```python
from build123d import *

# Parameters (mm, degrees)
ESQUISSE1_W             = 478.153686012
ESQUISSE1_H             = 188.593708553
ESQUISSE1_R             = 4
BOSS_EXTRU_4_DEPTH      = 5
ESQUISSE2_W             = 35.2
ESQUISSE2_H             = 34
ESQUISSE2_W_2           = 11
ENL_V_MAT_EXTRU_1_DEPTH = 2


with BuildPart() as part:
    # Esquisse1 → Boss.-Extru.4 (new body)
    with BuildSketch(Plane(origin=(0, 0, 0), x_dir=(1, 0, 0), z_dir=(0, 1, 0))):
        with Locations((166.159297522, 47.085285911)):
            Rectangle(ESQUISSE1_W, ESQUISSE1_H)
        with Locations(Location((395.236140528, -37.211568366, 0), (0, 0, 270))):
            Circle(ESQUISSE1_R, mode=Mode.SUBTRACT)
        with Locations(Location((-62.917545484, -37.211568366, 0), (0, 0, 270))):
            Circle(ESQUISSE1_R, mode=Mode.SUBTRACT)
        with Locations(Location((-32.917545484, -37.211568366, 0), (0, 0, 270))):
            Circle(ESQUISSE1_R, mode=Mode.SUBTRACT)
        with Locations(Location((365.236140528, -37.211568366, 0), (0, 0, 270))):
            Circle(ESQUISSE1_R, mode=Mode.SUBTRACT)
        with Locations(Location((-62.917545484, 131.382140187, 0), (0, 0, 270))):
            Circle(ESQUISSE1_R, mode=Mode.SUBTRACT)
        with Locations(Location((-32.917545484, 131.382140187, 0), (0, 0, 270))):
            Circle(ESQUISSE1_R, mode=Mode.SUBTRACT)
        with Locations(Location((365.236140528, 131.382140187, 0), (0, 0, 270))):
            Circle(ESQUISSE1_R, mode=Mode.SUBTRACT)
        with Locations(Location((395.236140528, 131.382140187, 0), (0, 0, 270))):
            Circle(ESQUISSE1_R, mode=Mode.SUBTRACT)
    extrude(amount=BOSS_EXTRU_4_DEPTH)

    # Esquisse2 → Enlèv. mat.-Extru.1 (cut)
    with BuildSketch(Plane(origin=(0, 5, 0), x_dir=(1, 0, 0), z_dir=(0, 1, 0))):
        with Locations((148.559297522, 122.382140187)):
            Rectangle(ESQUISSE2_W, ESQUISSE2_H)
        with Locations((171.659297522, 122.382140187)):
            Rectangle(ESQUISSE2_W_2, ESQUISSE2_H)
        with Locations((148.559297522, -28.211568366)):
            Rectangle(ESQUISSE2_W, ESQUISSE2_H)
        with Locations((171.659297522, -28.211568366)):
            Rectangle(ESQUISSE2_W_2, ESQUISSE2_H)
    extrude(amount=-ENL_V_MAT_EXTRU_1_DEPTH, mode=Mode.SUBTRACT)


solid = part.part
```
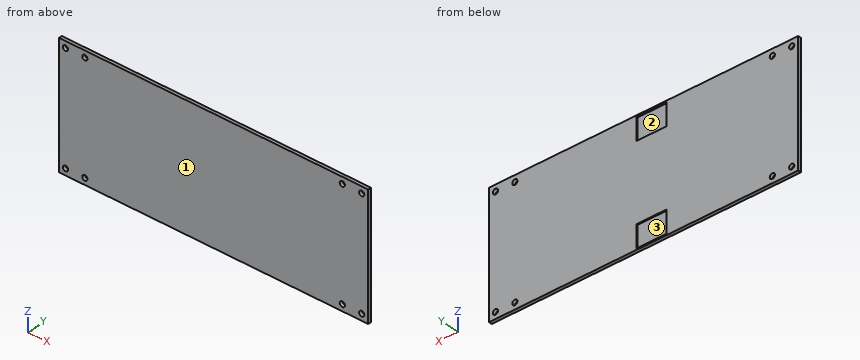
Here's how the part is built. I have some questions about the finished solid (model axes, mm). Face numbers are marked on the shaded views. Round coordinates to 2 decimals unless told otherwise and drop trailing zeros. Loops run counter-clockwise (first coordinate to the right, second up) from the corner with the lowest first, then second, coordinate; pieces in that order, holes last.
1. Will this pin go through, and if not, where does the flat tip stop? pin 1 (17 mm diameter, centred on x = 159.5, z = 35, fed in from +Y).
Answers:
pin 1: stops at y = 3
2. Suppose I cut it at B-B, the plane y = 4.05. Give the number of separate pieces and of enclosed holes in the cut face, and give its area (3 significant figures).
Answers:
separate pieces: 1
enclosed holes: 10
area: 86,600 mm2
3. If I drill on probe 1 along X at (y, z) = (3.25, -123.5); probe 2 along X at (y, z) = (1, -128), over which ranges is the centre line in solid material (lowest first)?
Answers:
probe 1: x = -72.92 to 130.96, 177.16 to 405.24
probe 2: x = -72.92 to -65.05, -60.78 to -35.05, -30.78 to 363.1, 367.37 to 393.1, 397.37 to 405.24
4. Suppose I cut it at A-A, the plane z = 27.5. Please give me the cut outline in (x, y).
Answers:
outline: (-72.92, 0) - (405.24, 0) - (405.24, 5) - (177.16, 5) - (177.16, 3) - (130.96, 3) - (130.96, 5) - (-72.92, 5) - close
5. Thinking about a two-plate mould opening in Z: for the marked faces 1, 2 and 3, which applies, released by +Z, released by -Z, zero draft, split by the parting line, or undercut?
Answers:
face 1: zero draft
face 2: undercut
face 3: undercut
